from build123d import *

# Parameters (mm, degrees)
SKETCH1_R                = 12
BOSS_EXTRUDE1_DEPTH      = 2
SKETCH2_R                = 1.5
BOSS_EXTRUDE2_DEPTH      = 2
SKETCH3_R                = 1.5
CUT_EXTRUDE1_DEPTH       = 5
SKETCH4_R                = 4
CUT_EXTRUDE2_DEPTH       = 2
SKETCH5_R                = 1.5
CUT_EXTRUDE3_DEPTH       = 2
SKETCH6_R                = 1.4
BOSS_EXTRUDE3_DEPTH      = 2
SKETCH7_R                = 1.6
CUT_EXTRUDE4_DEPTH       = 2
FILLET1_R                = 1
SKETCH8_R                = 4
BOSS_EXTRUDE7_DEPTH      = 5
SKETCH9_R                = 1.6
BOSS_EXTRUDE8_DEPTH      = 6
BOSS_EXTRUDE8_DEPTH_BACK = 2
SKETCH10_R               = 1.6
SKETCH10_R_2             = 1.495
CUT_EXTRUDE5_DEPTH       = 6
SKETCH11_R               = 4
BOSS_EXTRUDE9_DEPTH      = 2
CUT_EXTRUDE6_DEPTH       = 8
SKETCH13_R               = 6.833450219
CUT_EXTRUDE7_DEPTH       = 1
SKETCH14_R               = 7.033053892
CUT_EXTRUDE8_DEPTH       = 1
SKETCH15_R               = 8.776668046
CUT_EXTRUDE9_DEPTH       = 0.5
CUT_EXTRUDE10_DEPTH      = 2
CUT_EXTRUDE11_DEPTH      = 2


with BuildPart() as part:
    # Sketch1 → Boss-Extrude1 (new body)
    with BuildSketch(Plane(origin=(0, 0, 0), x_dir=(1, 0, 0), z_dir=(0, 1, 0))):
        Circle(SKETCH1_R)
    extrude(amount=BOSS_EXTRUDE1_DEPTH)

    # Sketch2 → Boss-Extrude2 (add)
    with BuildSketch(Plane(origin=(0, 2, 0), x_dir=(1, 0, 0), z_dir=(0, 1, 0))):
        with Locations((0, 9.5)):
            Circle(SKETCH2_R)
        with BuildLine():
            Line((-6, 0), (6, 0))
            ThreePointArc((6, 0), (0, -6), (-6, 0))
        make_face()
    extrude(amount=BOSS_EXTRUDE2_DEPTH)

    # Sketch3 → Cut-Extrude1 (cut)
    with BuildSketch(Plane.XZ):
        Circle(SKETCH3_R)
    extrude(amount=-CUT_EXTRUDE1_DEPTH, mode=Mode.SUBTRACT)

    # Sketch4 → Cut-Extrude2 (cut)
    with BuildSketch(Plane(origin=(0, 2, 0), x_dir=(1, 0, 0), z_dir=(0, 1, 0))):
        Circle(SKETCH4_R)
    extrude(amount=CUT_EXTRUDE2_DEPTH, mode=Mode.SUBTRACT)

    # Sketch5 → Cut-Extrude3 (cut)
    with BuildSketch(Plane(origin=(0, 2, 0), x_dir=(1, 0, 0), z_dir=(0, 1, 0))):
        with Locations((0, 9.5)):
            Circle(SKETCH5_R)
    extrude(amount=CUT_EXTRUDE3_DEPTH, mode=Mode.SUBTRACT)

    # Sketch6 → Boss-Extrude3 (add)
    with BuildSketch(Plane(origin=(0, 2, 0), x_dir=(1, 0, 0), z_dir=(0, 1, 0))):
        with Locations((0, 9.2)):
            Circle(SKETCH6_R)
    extrude(amount=BOSS_EXTRUDE3_DEPTH)

    # Sketch7 → Cut-Extrude4 (cut)
    with BuildSketch(Plane(origin=(0, 2, 0), x_dir=(1, 0, 0), z_dir=(0, 1, 0))):
        Circle(SKETCH7_R)
    extrude(amount=-CUT_EXTRUDE4_DEPTH, mode=Mode.SUBTRACT)

    # Fillet1
    fillet1_edges = [part.edges().sort_by_distance(p)[0] for p in [
        (-6, 3, 0),
        (6, 3, 0),
    ]]
    fillet(fillet1_edges, radius=FILLET1_R)

    # Sketch8 → Boss-Extrude7 (add)
    with BuildSketch(Plane(origin=(0, 0, 0), x_dir=(-1, 0, 0), z_dir=(0, -1, 0))):
        Circle(SKETCH8_R)
        with BuildLine():
            ThreePointArc((0.556776436, -1.5), (0, -1.6), (-0.556776436, -1.5))
            Line((-0.556776436, -1.5), (-2, -1.5))
            ThreePointArc((-2, -1.5), (-2.5, 0), (-2, 1.5))
            Line((-2, 1.5), (-0.556776436, 1.5))
            ThreePointArc((-0.556776436, 1.5), (0, 1.6), (0.556776436, 1.5))
            Line((0.556776436, 1.5), (2, 1.5))
            ThreePointArc((2, 1.5), (2.5, 0), (2, -1.5))
            Line((2, -1.5), (0.556776436, -1.5))
        make_face(mode=Mode.SUBTRACT)
    extrude(amount=BOSS_EXTRUDE7_DEPTH)

    # Sketch9 → Boss-Extrude8 (add, two sides)
    with BuildSketch(Plane(origin=(0, 2, 0), x_dir=(1, 0, 0), z_dir=(0, 1, 0))) as boss_extrude8_sk:
        Circle(SKETCH9_R)
    extrude(amount=BOSS_EXTRUDE8_DEPTH)
    extrude(boss_extrude8_sk.sketch, amount=-BOSS_EXTRUDE8_DEPTH_BACK)

    # Sketch10 → Cut-Extrude5 (cut)
    with BuildSketch(Plane(origin=(0, 8, 0), x_dir=(1, 0, 0), z_dir=(0, 1, 0))):
        Circle(SKETCH10_R)
        Circle(SKETCH10_R_2, mode=Mode.SUBTRACT)
    extrude(amount=-CUT_EXTRUDE5_DEPTH, mode=Mode.SUBTRACT)

    # Sketch11 → Boss-Extrude9 (add)
    with BuildSketch(Plane(origin=(0, 2, 0), x_dir=(1, 0, 0), z_dir=(0, 1, 0))):
        Circle(SKETCH11_R)
    extrude(amount=BOSS_EXTRUDE9_DEPTH)

    # Sketch12 → Cut-Extrude6 (cut)
    with BuildSketch(Plane(origin=(0, -5, 0), x_dir=(-1, 0, 0), z_dir=(0, -1, 0))):
        with BuildLine():
            Line((2, -1.5), (0.556776436, -1.5))
            ThreePointArc((0.556776436, -1.5), (0, -1.6), (-0.556776436, -1.5))
            Line((-0.556776436, -1.5), (-2, -1.5))
            ThreePointArc((-2, -1.5), (-2.5, 0), (-2, 1.5))
            Line((-2, 1.5), (-0.556776436, 1.5))
            ThreePointArc((-0.556776436, 1.5), (0, 1.6), (0.556776436, 1.5))
            Line((0.556776436, 1.5), (2, 1.5))
            ThreePointArc((2, 1.5), (2.5, 0), (2, -1.5))
        make_face()
    extrude(amount=-CUT_EXTRUDE6_DEPTH, mode=Mode.SUBTRACT)

    # Sketch13 → Cut-Extrude7 (cut)
    with BuildSketch(Plane(origin=(0, -5, 0), x_dir=(-1, 0, 0), z_dir=(0, -1, 0))):
        Circle(SKETCH13_R)
    extrude(amount=-CUT_EXTRUDE7_DEPTH, mode=Mode.SUBTRACT)

    # Sketch14 → Cut-Extrude8 (cut)
    with BuildSketch(Plane(origin=(0, -4, 0), x_dir=(-1, 0, 0), z_dir=(0, -1, 0))):
        Circle(SKETCH14_R)
    extrude(amount=-CUT_EXTRUDE8_DEPTH, mode=Mode.SUBTRACT)

    # Sketch15 → Cut-Extrude9 (cut)
    with BuildSketch(Plane(origin=(0, -3, 0), x_dir=(-1, 0, 0), z_dir=(0, -1, 0))):
        Circle(SKETCH15_R)
    extrude(amount=-CUT_EXTRUDE9_DEPTH, mode=Mode.SUBTRACT)

    # Sketch16 → Cut-Extrude10 (cut)
    with BuildSketch(Plane(origin=(0, 4, 0), x_dir=(1, 0, 0), z_dir=(0, 1, 0))):
        with BuildLine():
            Line((-4, 0), (-3, 0))
            ThreePointArc((-3, 0), (0, 3), (3, 0))
            Line((3, 0), (4, 0))
            Line((4, 0), (6.488398176, 5.447999119))
            Line((6.488398176, 5.447999119), (-6.411842689, 6.016687232))
            Line((-6.411842689, 6.016687232), (-4, 0))
        make_face()
    extrude(amount=-CUT_EXTRUDE10_DEPTH, mode=Mode.SUBTRACT)

    # Sketch17 → Cut-Extrude11 (cut)
    with BuildSketch(Plane(origin=(0, 4, 0), x_dir=(1, 0, 0), z_dir=(0, 1, 0))):
        with BuildLine():
            Line((-3, 0), (-2.5, 0))
            ThreePointArc((-2.5, 0), (0, 2.5), (2.5, 0))
            Line((2.5, 0), (3, 0))
            Line((3, 0), (3.695122569, 4.261417823))
            Line((3.695122569, 4.261417823), (-7.0808681, 5.499359859))
            Line((-7.0808681, 5.499359859), (-3, 0))
        make_face()
    extrude(amount=-CUT_EXTRUDE11_DEPTH, mode=Mode.SUBTRACT)


solid = part.part
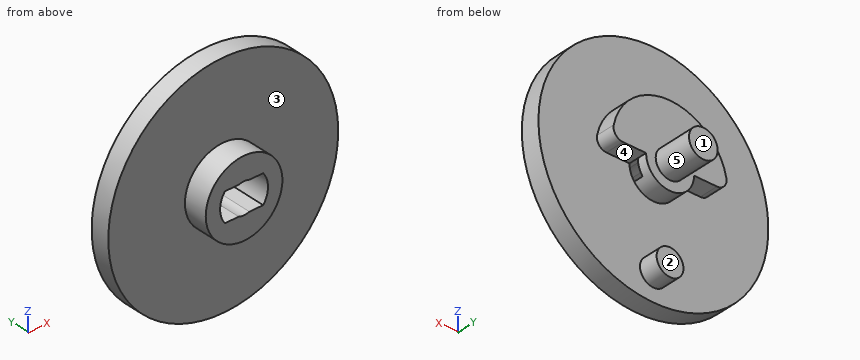
For this review, take the finished solid that the model builds, in its own axes (mm). Face numbers are marked on the shaded views. A direction names the side the tool comes from. Round coordinates to 2 decimals unless told otherwise and drop trailing zeros. Write each loop counter-clockwise with the first axis right and the second up, starting at its lowest first coordinate (ties: lowest second). Pieces come first, ordered by that corner, then holes. Notation, with made-up numbers: (1.25, 67.5) - (52.25, 67.5) arc R20 cw to (52.25, 71.5) - close; hole circle Ø6 at (88.25, 35.5). An arc over 180 degrees is marked (long way). Write item = value, one per line. Start each with the question number.
1. Consider section A-A on y = 3.5. State the section outline as (x, z) points, plus the area to 3 significant figures.
2. Wall thickness on L1, parallel to X at y = 6.75, z = 0 (3 decimals); L2, parallel to Y at x = -5, z = -9; L3, parallel to Y at x = -3.25, z = -0.25: over which ranges is each line inside the solid? List them lowest first.
3. For the marked faces 1, 2, 3, 4 and 5, list the 3-axis set-ups (+Z, -Z, +X, -X, +Y, -Y) from which the entire face can be reached by the end or side of a thin tool; tool diameter is ignored.
4. Consider section C-C on y = -0.5. State the section outline as (x, z) points.
5. For pin 1 Ø3 at (x, z) = (8, 1.5) entering from +Y; pin 2 Ø1.2 at (x, y) = (-1, 0) entering from +Z; pin 3 Ø4 at (y, z) = (5.5, -3) entering from -X, all flat-tipped, find the tip position at first contact; note any pin that passes through.
6. Consider section D-D on z = -9.2. State the section outline as (x, y) points, plus the area to 3 significant figures.
7. Consider section B-B on x = 0. State the section outline as (y, z) points (3 decimals), plus the area to 3 significant figures.
Evaluation:
q1.outline = (-5.88, 1.2) arc R1 ccw to (-4.9, 0) - (-2.5, 0) arc R2.5 ccw to (2.5, 0) - (4.9, 0) arc R1 ccw to (5.88, 1.2) arc R6 ccw to start; circle Ø2.8 at (0, -9.2)
q1.area = 71.9 mm2
q2.L1 = -1.495 to 1.495
q2.L2 = 0 to 2
q2.L3 = -2.5 to 2
q3.face_1 = +Z, -Z, +X, -X, +Y
q3.face_2 = -Z, +X, -X, +Y
q3.face_3 = -Y
q3.face_4 = -Z, +X, +Y
q3.face_5 = +Y
q4.outline = circle Ø8 at (0, 0); hole (-2, -1.5) - (-0.56, -1.5) arc R1.6 ccw to (0.56, -1.5) - (2, -1.5) arc R2.5 ccw to (2, 1.5) - (0.56, 1.5) arc R1.6 ccw to (-0.56, 1.5) - (-2, 1.5) arc R2.5 ccw to start
q5.pin_1 = 2
q5.pin_2 = 11.99
q5.pin_3 = -1.85
q6.outline = (-7.7, 0) - (7.7, 0) - (7.7, 2) - (1.4, 2) - (1.4, 4) - (-1.4, 4) - (-1.4, 2) - (-7.7, 2) - close
q6.area = 36.4 mm2
q7.outline = (-2.5, -4) - (0, -4) - (0, -12) - (2, -12) - (2, -10.6) - (4, -10.6) - (4, -7.8) - (2, -7.8) - (2, -2.5) - (4, -2.5) - (4, -1.495) - (8, -1.495) - (8, 1.495) - (4, 1.495) - (4, 6) - (2, 6) - (2, 12) - (0, 12) - (0, 4) - (-2.5, 4) - (-2.5, 1.6) - (3, 1.6) - (3, -1.6) - (-2.5, -1.6) - close
q7.area = 85.0 mm2
